Model file for the job. Use its own axes, mm. A direction names the side the tool comes from. Round coordinates to 2 decimals unless told otherwise and drop trailing zeros. Order: outer loops, then holes, each group sorted by start corner. A loop starts at its lowest first (then second) coordinate and runs counter-clockwise, first axis right, second up. Notation, with made-up numbers: (67, -7) - (93, -7) arc R24 ccw to (93, 13) - close; hole circle Ø8 at (-11.75, 82.5). An arc over 180 degrees is marked (long way). Write item = value, one per line. Start each with the question number.
from build123d import *

# Parameters (mm, degrees)
CROQUIS1_R              = 1.5
CROQUIS1_R_2            = 4
CROQUIS1_R_3            = 4.5
SALIENTE_EXTRUIR1_DEPTH = 6


with BuildPart() as part:
    # Croquis1 → Saliente-Extruir1 (new body)
    with BuildSketch(Plane.XY):
        with BuildLine():
            ThreePointArc((-141.730339063, 56.412363794), (-138.194805157, 57.876829888), (-136.730339063, 61.412363794))
            Line((-136.730339063, 61.412363794), (-136.730339063, 68.408394616))
            ThreePointArc((-136.730339063, 68.408394616), (-137.539641754, 71.135674591), (-139.705561488, 72.980076558))
            Line((-139.705561488, 72.980076558), (-165.141293909, 84.245449184))
            ThreePointArc((-165.141293909, 84.245449184), (-165.650008995, 84.506514587), (-166.12559145, 84.823953575))
            Line((-166.12559145, 84.823953575), (-243.282498112, 142.965853083))
            ThreePointArc((-243.282498112, 142.965853083), (-245.323514753, 145.031918552), (-246.684791002, 147.597323475))
            ThreePointArc((-246.684791002, 147.597323475), (-249.33333249, 155.226277836), (-253.46024382, 162.167770437))
            ThreePointArc((-253.46024382, 162.167770437), (-255.706791789, 164.36963499), (-258.526200935, 165.764668091))
            ThreePointArc((-258.526200935, 165.764668091), (-267.807267276, 167.484933762), (-277.233031605, 166.98246665))
            ThreePointArc((-277.233031605, 166.98246665), (-280.839635864, 165.006508056), (-281.744934312, 160.994969527))
            ThreePointArc((-281.744934312, 160.994969527), (-279.629843944, 151.795844616), (-275.418009863, 143.348480526))
            ThreePointArc((-275.418009863, 143.348480526), (-273.299883496, 141.022813744), (-270.564082899, 139.470209357))
            ThreePointArc((-270.564082899, 139.470209357), (-262.753961023, 137.416502238), (-254.690502443, 136.973385563))
            ThreePointArc((-254.690502443, 136.973385563), (-251.84925837, 136.371964278), (-249.300648344, 134.979497983))
            Line((-249.300648344, 134.979497983), (-172.090396499, 76.797399996))
            ThreePointArc((-172.090396499, 76.797399996), (-171.839715997, 76.595527407), (-171.602543042, 76.377944673))
            Line((-171.602543042, 76.377944673), (-152.656110988, 57.838641566))
            ThreePointArc((-152.656110988, 57.838641566), (-151.047487061, 56.782643978), (-149.159182416, 56.412363794))
            Line((-149.159182416, 56.412363794), (-141.730339063, 56.412363794))
        make_face()
        with Locations((-144.716694163, 62.430514025)):
            Circle(CROQUIS1_R, mode=Mode.SUBTRACT)
        with Locations((-162.290622468, 75.673418875)):
            Circle(CROQUIS1_R, mode=Mode.SUBTRACT)
        with Locations((-151.980339063, 71.662363794)):
            Circle(CROQUIS1_R_2, mode=Mode.SUBTRACT)
        with Locations((-180.655292115, 89.512190067)):
            Circle(CROQUIS1_R, mode=Mode.SUBTRACT)
        with BuildLine():
            Line((-271.680758131, 150.180525793), (-274.453508724, 149.79084111))
            ThreePointArc((-274.453508724, 149.79084111), (-276.147670478, 151.067483562), (-274.871028026, 152.761645316))
            Line((-274.871028026, 152.761645316), (-272.098277434, 153.151329999))
            ThreePointArc((-272.098277434, 153.151329999), (-270.404115679, 151.874687547), (-271.680758131, 150.180525793))
        make_face(mode=Mode.SUBTRACT)
        with Locations((-264.51202067, 152.702767498)):
            Circle(CROQUIS1_R_3, mode=Mode.SUBTRACT)
        with BuildLine():
            Line((-261.989778965, 145.534030037), (-261.600094282, 142.761279445))
            ThreePointArc((-261.600094282, 142.761279445), (-262.876736734, 141.06711769), (-264.570898489, 142.343760142))
            Line((-264.570898489, 142.343760142), (-264.960583171, 145.116510734))
            ThreePointArc((-264.960583171, 145.116510734), (-263.68394072, 146.810672489), (-261.989778965, 145.534030037))
        make_face(mode=Mode.SUBTRACT)
        with Locations((-274.894282301, 160.526362799)):
            Circle(CROQUIS1_R_2, mode=Mode.SUBTRACT)
        with BuildLine():
            Line((-267.034262376, 159.871504959), (-267.423947058, 162.644255551))
            ThreePointArc((-267.423947058, 162.644255551), (-266.147304607, 164.338417306), (-264.453142852, 163.061774854))
            Line((-264.453142852, 163.061774854), (-264.063458169, 160.289024262))
            ThreePointArc((-264.063458169, 160.289024262), (-265.340100621, 158.594862507), (-267.034262376, 159.871504959))
        make_face(mode=Mode.SUBTRACT)
        with BuildLine():
            Line((-257.34328321, 155.225009203), (-254.570532617, 155.614693886))
            ThreePointArc((-254.570532617, 155.614693886), (-252.876370863, 154.338051434), (-254.153013314, 152.64388968))
            Line((-254.153013314, 152.64388968), (-256.925763907, 152.254204997))
            ThreePointArc((-256.925763907, 152.254204997), (-258.619925661, 153.530847449), (-257.34328321, 155.225009203))
        make_face(mode=Mode.SUBTRACT)
    extrude(amount=SALIENTE_EXTRUIR1_DEPTH)


solid = part.part
Item 1: Saw through at A-A, the plane y = 66. Give the cut face in (x, z).
Item 2: Which spindle directions (+Z, -Z, +X, -X, +Y, -Y) get a long thin tool onto all of the face, cutting with end or side? Do faces 5 (the face through (-136.73, 65, 3)), 6 (the face through (-255.52, 152.45, 2.96)). Say none if no direction does.
Item 3: Saw through at B-B, the plane z = 2.55. Give the number of separate pieces and of enclosed holes in the cut face, then the cut area to 3 significant figures.
Item 4: Saw through at C-C, the plane x = -227. Give the cut face in (y, z).
Item 5: Probe L1, parallel to Y at x = -274, z = 2.7; L2, parallel to Y at x = -161.5, z = 3.85; L3, parallel to X at y = 62, z = 4.3. List the from-to ranges inside material, lowest first.
Item 6: Drop flat-ended pins along their axis: pin 1 (2 mm diameter, centred on y = 89.5, z = 4.5, fed in from +X); pin 2 (3 mm diameter, centred on x = -224.5, z = 4.5, fed in from +Y); pin 3 (3.5 mm diameter, centred on x = -144.72, y = 62.43, fed in from -Z); pin 4 (3 mm diameter, centred on x = -245.5, z = 4.5, fed in from -Y). Give the stop position or say it passes through.
Item 7: Mould opens along X. For faces 1 (the face through (-138.23, 57.84, 2.96)), 2 (the face through (-145, 56.412, 3)), 3 (the face through (-211.24, 106.3, 2.96)), 4 (the face through (-275.76, 156.62, 2.96)) say: +X half, -X half, draft (parallel to the pull), parting line (faces both ways), or undercut.
Check sheet entries:
q1.outline = (-161, 0) - (-136.73, 0) - (-136.73, 6) - (-161, 6) - close
q2.face_5 = +Z, -Z, +X, +Y, -Y
q2.face_6 = +Z, -Z
q3.separate_pieces = 1
q3.enclosed_holes = 10
q3.area = 2,150 mm2
q4.outline = (118.17, 0) - (130.7, 0) - (130.7, 6) - (118.17, 6) - close
q5.L1 = 141.64 to 149.85, 152.88 to 156.63, 164.43 to 167.41
q5.L2 = 66.49 to 74.4, 76.95 to 82.63
q5.L3 = -156.91 to -146.15, -143.28 to -136.73
q6.pin_1 = -171
q6.pin_2 = 129.94
q6.pin_3 = 0
q6.pin_4 = 130.99
q7.face_1 = +X half
q7.face_2 = draft
q7.face_3 = -X half
q7.face_4 = undercut
